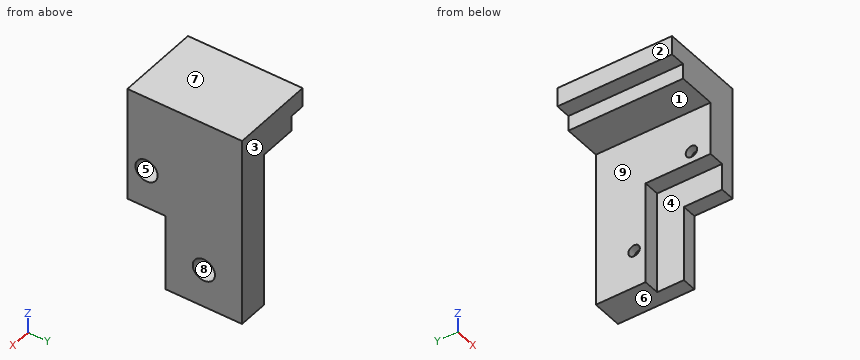
from build123d import *

# Parameters (mm, degrees)
SKETCH_1_W           = 40
SKETCH_1_H           = 30
EXTRUDE_1_DEPTH      = 5
SKETCH_2_W           = 5
SKETCH_2_H           = 30
EXTRUDE_2_DEPTH      = 20
SKETCH_3_W           = 20
SKETCH_3_H           = 30
EXTRUDE_3_DEPTH      = 5
SKETCH_4_W           = 15
SKETCH_4_H           = 30
CUT_EXTRUDE_1_DEPTH  = 5
SKETCH_6_R           = 1.5
CUT_EXTRUDE_3_DEPTH  = 5
SKETCH_7_W           = 15
SKETCH_7_H           = 30
CUT_EXTRUDE_4_DEPTH  = 5
SKETCH_8_W           = 5
SKETCH_8_H           = 30
EXTRUDE_4_DEPTH      = 20
SKETCH_9_W           = 30
SKETCH_9_H           = 30
EXTRUDE_5_DEPTH      = 3
SKETCH_10_R          = 1.5
CUT_EXTRUDE_5_DEPTH  = 13
SKETCH_11_R          = 2.9
CUT_EXTRUDE_6_DEPTH  = 6
SKETCH_12_W          = 8
SKETCH_12_H          = 20
EXTRUDE_6_DEPTH      = 20
CUT_EXTRUDE_7_DEPTH  = 4.2
SKETCH_14_R          = 1.5
CUT_EXTRUDE_8_DEPTH  = 14.2
SKETCH_15_R          = 2.9
CUT_EXTRUDE_9_DEPTH  = 6
SKETCH_16_W          = 4
SKETCH_16_H          = 30
EXTRUDE_7_DEPTH      = 9.95
SKETCH_17_W          = 5
SKETCH_17_H          = 30
CUT_EXTRUDE_10_DEPTH = 26.05


with BuildPart() as part:
    # 草图1 → 凸台-拉伸1 (new body)
    with BuildSketch(Plane.XY):
        with Locations((-20, 15)):
            Rectangle(SKETCH_1_W, SKETCH_1_H)
    extrude(amount=EXTRUDE_1_DEPTH)

    # 草图2 → 凸台-拉伸2 (add)
    with BuildSketch(Plane.ZY.offset(40)):
        with Locations((2.5, 15)):
            Rectangle(SKETCH_2_W, SKETCH_2_H)
    extrude(amount=EXTRUDE_2_DEPTH)

    # 草图3 → 凸台-拉伸3 (add)
    with BuildSketch(Plane(origin=(0, 0, 0), x_dir=(-1, 0, 0), z_dir=(0, 0, -1))):
        with Locations((10, 15)):
            Rectangle(SKETCH_3_W, SKETCH_3_H)
    extrude(amount=EXTRUDE_3_DEPTH)

    # 草图4 → 切除-拉伸1 (cut)
    with BuildSketch(Plane.XY.offset(5)):
        with Locations((-7.5, 15)):
            Rectangle(SKETCH_4_W, SKETCH_4_H)
    extrude(amount=-CUT_EXTRUDE_1_DEPTH, mode=Mode.SUBTRACT)

    # 草图6 → 切除-拉伸3 (cut)
    with BuildSketch(Plane.XY):
        with Locations((-7.5, 25)):
            Circle(SKETCH_6_R)
        with Locations((-7.5, 5)):
            Circle(SKETCH_6_R)
    extrude(amount=-CUT_EXTRUDE_3_DEPTH, mode=Mode.SUBTRACT)

    # 草图7 → 切除-拉伸4 (cut)
    with BuildSketch(Plane.XY):
        with Locations((-7.5, 15)):
            Rectangle(SKETCH_7_W, SKETCH_7_H)
    extrude(amount=-CUT_EXTRUDE_4_DEPTH, mode=Mode.SUBTRACT)

    # 草图8 → 凸台-拉伸4 (add)
    with BuildSketch(Plane(origin=(0, 0, -5), x_dir=(-1, 0, 0), z_dir=(0, 0, -1))):
        with Locations((17.5, 15)):
            Rectangle(SKETCH_8_W, SKETCH_8_H)
    extrude(amount=EXTRUDE_4_DEPTH)

    # 草图9 → 凸台-拉伸5 (add)
    with BuildSketch(Plane(origin=(-15, 0, 0), x_dir=(0, 0, -1), z_dir=(1, 0, 0))):
        with Locations((10, 15)):
            Rectangle(SKETCH_9_W, SKETCH_9_H)
    extrude(amount=EXTRUDE_5_DEPTH)

    # 草图10 → 切除-拉伸5 (cut)
    with BuildSketch(Plane(origin=(-12, 0, 0), x_dir=(0, 0, -1), z_dir=(1, 0, 0))):
        with Locations((15, 5)):
            Circle(SKETCH_10_R)
    extrude(amount=-CUT_EXTRUDE_5_DEPTH, mode=Mode.SUBTRACT)

    # 草图11 → 切除-拉伸6 (cut)
    with BuildSketch(Plane(origin=(-12, 0, 0), x_dir=(0, 0, -1), z_dir=(1, 0, 0))):
        with Locations((15, 5)):
            Circle(SKETCH_11_R)
    extrude(amount=-CUT_EXTRUDE_6_DEPTH, mode=Mode.SUBTRACT)

    # 草图12 → 凸台-拉伸6 (add)
    with BuildSketch(Plane(origin=(0, 0, -25), x_dir=(-1, 0, 0), z_dir=(0, 0, -1))):
        with Locations((16, 20)):
            Rectangle(SKETCH_12_W, SKETCH_12_H)
    extrude(amount=EXTRUDE_6_DEPTH)

    # 草图13 → 切除-拉伸7 (cut)
    with BuildSketch(Plane.ZY.offset(20)):
        Polygon((-45, 17), (-25, 17), (-18, 17), (-18, 0), (-25, 0), (-25, 10), (-45, 10), align=None)
    extrude(amount=-CUT_EXTRUDE_7_DEPTH, mode=Mode.SUBTRACT)

    # 草图14 → 切除-拉伸8 (cut)
    with BuildSketch(Plane(origin=(-12, 0, 0), x_dir=(0, 0, -1), z_dir=(1, 0, 0))):
        with Locations((35, 20)):
            Circle(SKETCH_14_R)
    extrude(amount=-CUT_EXTRUDE_8_DEPTH, mode=Mode.SUBTRACT)

    # 草图15 → 切除-拉伸9 (cut)
    with BuildSketch(Plane(origin=(-12, 0, 0), x_dir=(0, 0, -1), z_dir=(1, 0, 0))):
        with Locations((35, 20)):
            Circle(SKETCH_15_R)
    extrude(amount=-CUT_EXTRUDE_9_DEPTH, mode=Mode.SUBTRACT)

    # 草图16 → 凸台-拉伸7 (add)
    with BuildSketch(Plane.ZY.offset(20)):
        with Locations((-2, 15)):
            Rectangle(SKETCH_16_W, SKETCH_16_H)
    extrude(amount=EXTRUDE_7_DEPTH)

    # 草图17 → 切除-拉伸10 (cut)
    with BuildSketch(Plane.ZY.offset(60)):
        with Locations((2.5, 15)):
            Rectangle(SKETCH_17_W, SKETCH_17_H)
    extrude(amount=-CUT_EXTRUDE_10_DEPTH, mode=Mode.SUBTRACT)


solid = part.part
Build history of the part. All positions in model axes, mm. Face numbers are marked on the shaded views. A direction names the side the tool comes from. Round coordinates to 2 decimals unless told otherwise and drop trailing zeros. Write each loop counter-clockwise with the first axis right and the second up, starting at its lowest first coordinate (ties: lowest second). Pieces come first, ordered by that corner, then holes. Notation, with made-up numbers: M 50.25,64 L 100.25,64 A12 cw 100.25,69 Z; hole C 26.25,-13 d1. An arc over 180 degrees is marked long. Answer in a Markdown table with one row per item.
1. Saw through at D-D (z = -15). List the corners of the cut face in (x, y).
Geometry check:
| item | result |
|---|---|
| outline | M -20,0 L -12,0 L -12,2.1 L -18,2.1 L -18,3.5 L -20,3.5 Z; M -20,6.5 L -18,6.5 L -18,7.9 L -12,7.9 L -12,30 L -20,30 Z |
2. Which spindle directions (+Z, -Z, +X, -X, +Y, -Y) get a long thin tool onto all of the face, cutting with end or side? Do the marked faces 1, 2, 3, 4 and 5. Say none if no direction does.
Geometry check:
| item | result |
|---|---|
| face 1 | -Z, -X, +Y, -Y |
| face 2 | +Z, -Z, -X, +Y, -Y |
| face 3 | +Z, -Z, +X, -X, +Y |
| face 4 | -Z, -X, -Y |
| face 5 | +X |
3. Mould opens along Z. For the marked faces 6, 7, 8 and 9 say: +Z half, -Z half, draft (parallel to the pull), parting line (faces both ways), or undercut.
Geometry check:
| item | result |
|---|---|
| face 6 | -Z half |
| face 7 | +Z half |
| face 8 | undercut |
| face 9 | draft |
4. Probe L1, parallel to Y at x = -18.4, z = -35; L2, parallel to Y at x = -18.85, z = -15; L3, parallel to Z at x = -22.5, y = 27. List the from-to ranges inside material, lowest first. Write a range as [from, to].
Geometry check:
| item | result |
|---|---|
| L1 | [17, 18.5], [21.5, 30] |
| L2 | [0, 3.5], [6.5, 30] |
| L3 | [-4, 5] |
5. Saw through at B-B (y = 20). List the corners of the cut face in (x, z).
Geometry check:
| item | result |
|---|---|
| outline | M -33.95,0 L -29.95,0 L -29.95,-4 L -20,-4 L -20,-33.5 L -18,-33.5 L -18,-32.1 L -12,-32.1 L -12,5 L -33.95,5 Z; M -20,-45 L -12,-45 L -12,-37.9 L -18,-37.9 L -18,-36.5 L -20,-36.5 Z |
6. Saw through at C-C (x = -14.5). List the corners of the cut face in (y, z), and give its area (3 significant figures).
Geometry check:
| item | result |
|---|---|
| outline | M 0,-25 L 10,-25 L 10,-45 L 30,-45 L 30,5 L 0,5 Z; hole C 5,-15 d5.8; hole C 20,-35 d5.8 |
| area | 1,250 mm2 |
7. Flat gauge pins, fed straight in: P1, Ø1.2, axis at x = -31, y = 22, coming from the -Z side; P2, Ø3, axis at x = -22.5, z = -12.5, coming from the -Y side; P3, Ø11, axis at x = -24.5, y = 20.5, coming from the -Z side; P4, Ø1.3, axis at x = -18, y = 8, coming from the -Z side. Where does each tip first touch, or does it go through?
Geometry check:
| item | result |
|---|---|
| P1 | z = 0 |
| P2 | through |
| P3 | z = -45 |
| P4 | z = -18 |
8. Saw through at A-A (z = -35). List the corners of the cut face in (x, y), and give its area (3 significant figures).
Geometry check:
| item | result |
|---|---|
| outline | M -20,17 L -15.8,17 L -15.8,10 L -12,10 L -12,17.1 L -18,17.1 L -18,18.5 L -20,18.5 Z; M -20,21.5 L -18,21.5 L -18,22.9 L -12,22.9 L -12,30 L -20,30 Z |
| area | 89.8 mm2 |
